from build123d import *

# Parameters (mm, degrees)
STOCK_BEE_ZERKER_START                       = 34.925
STOCK_BEE_ZERKER_2_0_MULTIBODY_1_OUTLINE_R   = 2.38125
STOCK_BEE_ZERKER_2_0_MULTIBODY_1_OUTLINE_R_2 = 3.175
STOCK_BEE_ZERKER_2_0_MULTIBODY_1_DEPTH       = 6.35
FILLET1_R                                    = 0.635
FILLET2_R                                    = 25.4


# Read off the part's stored shape, not the designer's step: Stock-Bee-zerker 2.0 Multibody-1
with BuildPart() as part:
    # Stock-Bee-zerker 2.0 Multibody-1 outline → Stock-Bee-zerker 2.0 Multibody-1 (new body)
    with BuildSketch(Plane.YZ.offset(STOCK_BEE_ZERKER_START)):
        Polygon((9.525, 108.397291582), (0, 128.82372), (0, 64.1985), (0.762, 38.33622), (2.286, 38.33622), (2.286, 39.92372), (30.58384403, 39.92372), (6.35, 68.804490685), (6.35, 108.957129746), align=None)
        with Locations((7.233375897, 55.251985719)):
            Circle(STOCK_BEE_ZERKER_2_0_MULTIBODY_1_OUTLINE_R, mode=Mode.SUBTRACT)
        with Locations((10.414, 46.27372)):
            Circle(STOCK_BEE_ZERKER_2_0_MULTIBODY_1_OUTLINE_R_2, mode=Mode.SUBTRACT)
    extrude(amount=STOCK_BEE_ZERKER_2_0_MULTIBODY_1_DEPTH)

    # Fillet1
    fillet1_edges = [part.edges().sort_by_distance(p)[0] for p in [
        (38.1, 6.35, 108.957129746),
        (38.1, 30.58384403, 39.92372),
        (38.1, 2.286, 39.92372),
        (38.1, 2.286, 38.33622),
        (38.1, 0.762, 38.33622),
    ]]
    fillet(fillet1_edges, radius=FILLET1_R)

    # Fillet2
    # the kernel refuses this fillet: 25.4 mm, written as the material it adds along each edge
    with BuildSketch(Plane(origin=(34.925, 6.35, 68.804490685), x_dir=(0, 0, 1), z_dir=(1, 0, 0))) as fillet2_piece_1:
        with BuildLine():
            CenterArc((FILLET2_R * 0.363970234267, -FILLET2_R), FILLET2_R, 90, 40)
            Line((-FILLET2_R * 0.278817375421, -FILLET2_R * 0.233955556882), (0, 0))
            Line((0, 0), (FILLET2_R * 0.363970234267, 0))
        make_face()
    extrude(amount=6.35)
    # the kernel refuses this fillet: 25.4 mm, written as the material it takes off along each edge
    with BuildSketch(Plane(origin=(33.98972857, 0, 64.1985), x_dir=(0, 0.029450978958150506, -0.9995662258391919), z_dir=(1, 0, 0))) as fillet2_2_piece_1:
        with BuildLine():
            CenterArc((FILLET2_R * 0.0147286839403, FILLET2_R), FILLET2_R, 268.312339175, 1.687660825)
            Line((-FILLET2_R * 0.0147222950178, FILLET2_R * 0.000433774160808), (0, 0))
            Line((0, 0), (FILLET2_R * 0.0147286839403, 0))
        make_face()
    extrude(amount=8.22054286, mode=Mode.SUBTRACT)


solid = part.part
Geometry check sheet. Reference: the model listing, model coordinates, mm. A direction names the side the tool comes from. Round coordinates to 2 decimals unless told otherwise and drop trailing zeros. Loops run counter-clockwise (first coordinate to the right, second up) from the corner with the lowest first, then second, coordinate; pieces in that order, holes last.
Item 1: Thickness scan on line 1 (Z direction, x = 35.5, y = 8.75); line 2 (Y direction, x = 37.5, z = 80); line 3 (Y direction, x = 40.25, z = 45). Record the ranges inside material, lowest first.
Item 2: Cross-section at B-B on z = 92. Record the boundary of the cut face in (x, y) (3 decimals).
Item 3: Gauge pin test, flat ends, axial feed: pin 1 (1.9 mm diameter, centred on x = 37, z = 95, fed in from +Y); pin 2 (7.5 mm diameter, centred on y = 10.41, z = 46.27, fed in from +X) (3 decimals); pin 3 (2 mm diameter, centred on x = 39, y = 5, fed in from -Z); pin 4 (2 mm diameter, centred on x = 40.5, z = 47.5, fed in from +Y). Record the tip position at first contact, or that the pin passes through.
Item 4: Cross-section at C-C on y = 21.25. Record the boundary of the cut face in (x, z) (3 decimals), then the cut area to 3 significant figures.
Item 5: Access from +Z, -Z, +X, -X, +Y, -Y to the whole of each face (thin tool, end or side, straight path). Record for faces 5 (the flat face through (38, 16, 39.924)), 6 (the flat face through (38.056, 8.293, 108.615)), 7 (the flat face through (41.275, 6, 70)), 8 (the cylindrical face through (38.06, 7.84, 69.48)).
Item 6: Cross-section at A-A on x = 39.25. Count the separate pieces of the cut face and the enclosed holes in it, then the cut area to 3 significant figures.
Item 7: Mould release check, pull along Z, two halves, no side actions. Record for faces 1 (the flat face through (38, 6.35, 93)), 2 (the cylindrical face through (38.06, 10, 49.42)), 3 (the flat face through (38.06, 4.83, 118.47)), 4 (the flat face through (38, 0, 97)): pulls with the +Z half, pulls with the -Z half, needs draft (parallel to the pull), parting line crosses it, or undercut.
Answer sheet:
1. line 1: z = 39.92 to 43.57, 48.98 to 53.42, 57.09 to 67.27, 108.53 to 110.06
1. line 2: y = 0 to 6.35
1. line 3: y = 0.57 to 7.51, 13.32 to 26.32
2. outline: (34.925, 0) - (41.275, 0) - (41.275, 6.35) - (34.925, 6.35) - close
3. pin 1: stops at y = 6.35
3. pin 2: stops at x = 41.275
3. pin 3: stops at z = 39.92
3. pin 4: stops at y = 25.07
4. outline: (34.925, 39.924) - (41.275, 39.924) - (41.275, 51.047) - (34.925, 51.047) - close
4. area: 70.6 mm2
5. face 5: -Z, +X, -X, +Y
5. face 6: +X, -X
5. face 7: +Z, -Z, +X, +Y, -Y
5. face 8: +X, -X, +Y
6. separate pieces: 1
6. enclosed holes: 2
6. area: 835 mm2
7. face 1: undercut
7. face 2: undercut
7. face 3: pulls with the +Z half
7. face 4: needs draft
